Geometry check sheet. Reference: the model listing, model coordinates, mm. Give positions to 0.01 mm unless a question says otherwise; leave off trailing zeros. Loops run counter-clockwise (first coordinate to the right, second up) from the corner with the lowest first, then second, coordinate; pieces in that order, holes last. Notation, with made-up numbers: (67, -8.75) - (73, -8.75) arc R18 cw to (73, -1.75) - close; hole circle Ø2 at (47.25, 79). An arc over 180 degrees is marked (long way). One line per question, with ' | ' between items. Start each with the question number.
from build123d import *

# Parameters (mm, degrees)
SKETCH1_W           = 19
SKETCH1_H           = 58
BOSS_EXTRUDE1_DEPTH = 54
SKETCH2_3_R         = 20
SKETCH2_3_R_2       = 15.5
BOSS_EXTRUDE2_DEPTH = 50
SKETCH2_R           = 1.9
CUT_EXTRUDE1_DEPTH  = 10
FILLET1_R           = 10
BOSS_EXTRUDE3_DEPTH = 50
SKETCH4_R           = 1.25
CUT_EXTRUDE2_DEPTH  = 55
SKETCH5_W           = 17
SKETCH5_H           = 14
CUT_EXTRUDE3_DEPTH  = 2
SKETCH7_W           = 50
SKETCH7_H           = 57
CUT_EXTRUDE4_DEPTH  = 59
SKETCH8_W           = 3
SKETCH8_H           = 14
BOSS_EXTRUDE4_DEPTH = 10
FILLET2_R           = 5


with BuildPart() as part:
    # Sketch1 → Boss-Extrude1 (new body)
    with BuildSketch(Plane.XY):
        with Locations((9.5, 29)):
            Rectangle(SKETCH1_W, SKETCH1_H)
    extrude(amount=BOSS_EXTRUDE1_DEPTH)

    # Sketch2_3 → Boss-Extrude2 (add)
    with BuildSketch(Plane.ZY):
        with Locations((27.5, 29)):
            Circle(SKETCH2_3_R)
        with Locations((27.5, 29)):
            Circle(SKETCH2_3_R_2, mode=Mode.SUBTRACT)
    extrude(amount=-BOSS_EXTRUDE2_DEPTH)

    # Sketch2 → Cut-Extrude1 (cut)
    with BuildSketch(Plane.ZY):
        with Locations((9.25, 29)):
            Circle(SKETCH2_R)
        with Locations((45.75, 29)):
            Circle(SKETCH2_R)
    extrude(amount=-CUT_EXTRUDE1_DEPTH, mode=Mode.SUBTRACT)

    # Fillet1
    fillet1_edges = [part.edges().sort_by_distance(p)[0] for p in [
        (9.5, 0, 0),
    ]]
    fillet(fillet1_edges, radius=FILLET1_R)

    # Sketch3 → Boss-Extrude3 (add)
    with BuildSketch(Plane(origin=(0, 0, 0), x_dir=(0, 0, -1), z_dir=(1, 0, 0))):
        Polygon((0, 0), (0, 57), (0, 67), (-5, 67), (-5, 0), align=None)
    extrude(amount=-BOSS_EXTRUDE3_DEPTH)

    # Sketch4 → Cut-Extrude2 (cut, through all)
    with BuildSketch(Plane(origin=(0, 0, 0), x_dir=(-1, 0, 0), z_dir=(0, 0, -1))):
        with Locations((14, 57)):
            Circle(SKETCH4_R)
        Polygon((0, 53), (0, 0), (50, 0), (50, 67), (17, 67), (17, 53), align=None)
        with Locations((14, 63.5)):
            Circle(SKETCH4_R)
    extrude(amount=-CUT_EXTRUDE2_DEPTH, mode=Mode.SUBTRACT)

    # Sketch5 → Cut-Extrude3 (cut)
    with BuildSketch(Plane(origin=(0, 0, 0), x_dir=(-1, 0, 0), z_dir=(0, 0, -1))):
        with Locations((8.5, 60)):
            Rectangle(SKETCH5_W, SKETCH5_H)
    extrude(amount=-CUT_EXTRUDE3_DEPTH, mode=Mode.SUBTRACT)

    # Sketch7 → Cut-Extrude4 (cut, through all)
    with BuildSketch(Plane(origin=(0, 58, 0), x_dir=(1, 0, 0), z_dir=(0, 1, 0))):
        with Locations((25, -28.5)):
            Rectangle(SKETCH7_W, SKETCH7_H)
    extrude(amount=-CUT_EXTRUDE4_DEPTH, mode=Mode.SUBTRACT)

    # Sketch8 → Boss-Extrude4 (add)
    with BuildSketch(Plane(origin=(0, 0, 0), x_dir=(0, 0, -1), z_dir=(1, 0, 0))):
        with Locations((-3.5, 60)):
            Rectangle(SKETCH8_W, SKETCH8_H)
    extrude(amount=BOSS_EXTRUDE4_DEPTH)

    # Fillet2
    fillet2_edges = [part.edges().sort_by_distance(p)[0] for p in [
        (10, 67, 3.5),
    ]]
    fillet(fillet2_edges, radius=FILLET2_R)


solid = part.part
(1) Section check C-C, the plane z = 2.9. Record the boundary of the cut face in (x, y).
(2) Depth check by flat-ended pin: pin 1 Ø4 at (x, y) = (-14, 57) entering from +Z. Enter the tip coordinate at first touch or a pass-through.
(3) Mould release check, pull along Y, two halves, no side actions. Record for faces 1 (the face through (-4, 60, 5)), 2 (the face through (8, 66, 3)), 3 (the face through (-13.84, 58.24, 3.48)), 4 (the face through (-13.84, 64.74, 3.48)): pulls with the +Y half, pulls with the -Y half, needs draft (parallel to the pull), parting line crosses it, or undercut.
(4) Material ranges on line 1 (Y direction, x = -14, z = 3.8); line 2 (X direction, y = 62.75, z = 2.7); line 3 (X direction, y = 57.5, z = 4.8), recorded low to high.
(5) Section check D-D, the plane y = 57. Record the boundary of the cut face in (x, z), and give its area (3 significant figures).
(6) Section check A-A, the plane y = 63.5. Record the boundary of the cut face in (x, z).
(7) Section check B-B, the plane x = -14. Record the boundary of the cut face in (y, z), and give its area (3 significant figures).
Numbers:
1) outline: (-17, 53) - (10, 53) - (10, 62) arc R5 ccw to (5, 67) - (-17, 67) - close; hole circle Ø2.5 at (-14, 57); hole circle Ø2.5 at (-14, 63.5)
2) pin 1: z = 5
3) face 1: needs draft | face 2: pulls with the +Y half | face 3: undercut | face 4: undercut
4) line 1: 53 to 55.75, 58.25 to 62.25, 64.75 to 67 | line 2: -17 to -15, -13 to 9.94 | line 3: -17 to -15.15, -12.85 to 10
5) outline: (-17, 2) - (-15.25, 2) - (-15.25, 5) - (-17, 5) - close; (-12.75, 2) - (10, 2) - (10, 5) - (-12.75, 5) - close | area: 73.5 mm^2
6) outline: (-17, 2) - (-15.25, 2) - (-15.25, 5) - (-17, 5) - close; (-12.75, 2) - (9.77, 2) - (9.77, 5) - (-12.75, 5) - close
7) outline: (53, 2) - (55.75, 2) - (55.75, 5) - (53, 5) - close; (58.25, 2) - (62.25, 2) - (62.25, 5) - (58.25, 5) - close; (64.75, 2) - (67, 2) - (67, 5) - (64.75, 5) - close | area: 27.0 mm^2
